```python
from build123d import *

# Parameters (mm, degrees)
BOSS_EXTRUDE2_DEPTH      = 7.35
BOSS_EXTRUDE2_DEPTH_BACK = 7.35
SKETCH2_W                = 15.7
SKETCH2_H                = 15.7
SKETCH3_R                = 8
BOSS_EXTRUDE3_DEPTH      = 20.55
SKETCH4_R                = 7.55
BOSS_EXTRUDE4_DEPTH      = 25.9
BOSS_EXTRUDE5_DEPTH      = 10
SKETCH6_R                = 8
BOSS_EXTRUDE6_DEPTH      = 20.55


with BuildPart() as part:
    # Sketch2 → Boss-Extrude2 (new, two sides: drawn at the far end of the back side and taken through both)
    with BuildSketch(Plane(origin=(0, 0, 0), x_dir=(1, 0, 0), z_dir=(0, 1, 0)).offset(-BOSS_EXTRUDE2_DEPTH_BACK)):
        Rectangle(SKETCH2_W, SKETCH2_H)
    extrude(amount=BOSS_EXTRUDE2_DEPTH + BOSS_EXTRUDE2_DEPTH_BACK)

    # Sketch3 → Boss-Extrude3 (add)
    with BuildSketch(Plane(origin=(7.85, 0, 0), x_dir=(0, 0, -1), z_dir=(1, 0, 0))):
        with Locations(Location((-0.75, 0, 0), (0, 0, 152.560759849))):
            Circle(SKETCH3_R)
    extrude(amount=BOSS_EXTRUDE3_DEPTH)

    # Sketch4 → Boss-Extrude4 (add)
    with BuildSketch(Plane(origin=(0, 0, -7.85), x_dir=(-1, 0, 0), z_dir=(0, 0, -1))):
        with Locations(Location((0, 0, 0), (0, 0, 103.217293988))):
            Circle(SKETCH4_R)
    extrude(amount=BOSS_EXTRUDE4_DEPTH)

    # Sketch5 → Boss-Extrude5 (add)
    with BuildSketch(Plane(origin=(0, 0, -33.75), x_dir=(-1, 0, 0), z_dir=(0, 0, -1))):
        Polygon((-15.532193585, 0), (-10.572107213, -10.198544939), (25.717504309, -7.313596743), (28.4, 0), (25.717504309, 7.313596743), (-10.572107213, 10.198544939), align=None)
    extrude(amount=-BOSS_EXTRUDE5_DEPTH)

    # Sketch6 → Boss-Extrude6 (add)
    with BuildSketch(Plane.XY.offset(7.85)):
        with Locations(Location((0, 0, 0), (0, 0, 168.887310083))):
            Circle(SKETCH6_R)
    extrude(amount=BOSS_EXTRUDE6_DEPTH)


solid = part.part
```
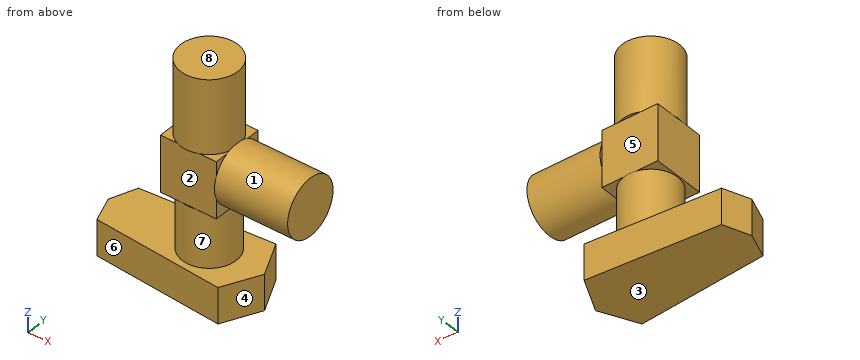
Verification items for the finished model (mm, model axes). Face numbers are marked on the shaded views. A direction names the side the tool comes from. Coordinates: 2 decimals unless noted, no trailing zeros. Loops run counter-clockwise (first coordinate to the right, second up) from the corner with the lowest first, then second, coordinate; pieces in that order, holes last. Notation, with made-up numbers: (-37.75, 80.5) -> (6.25, 80.5) arc R29 ccw to (6.25, 109.5) -> close; hole circle Ø2 at (-34, 26.25). An arc over 180 degrees is marked (long way). Put each result on its own line as item: value.
1. Gauge pin test, flat ends, axial feed: P1, Ø2, axis at x = 11, z = 1.5, coming from the -Y side; P2, Ø12, axis at y = 2, z = 2.5, coming from the -X side; P3, Ø10, axis at x = 19, z = -6.5, coming from the -Y side; P4, Ø8, axis at y = 3, z = -7.5, coming from the +X side. Record the tip position at first contact, or that the pin passes through.
Result set:
P1: stops at y = -8
P2: stops at x = -8
P3: stops at y = -7.68
P4: stops at x = 28.4
2. Section check D-D, the plane z = 13.5. Record the boundary of the cut face in (x, y).
Result set:
outline: circle Ø16 at (0, 0)
3. Mould release check, pull along Z, two halves, no side actions. Record for the marked faces 6, 7 and 8: pulls with the +Z half, pulls with the -Z half, needs draft (parallel to the pull), parting line crosses it, or undercut.
Result set:
face 6: needs draft
face 7: undercut
face 8: pulls with the +Z half
4. Section check C-C, the plane y = 8.75. Record the boundary of the cut face in (x, z).
Result set:
outline: (-7.65, -33.75) -> (11.28, -33.75) -> (11.28, -23.75) -> (-7.65, -23.75) -> close
5. Tool access check on the marked faces 1, 2, 3, 4 and 5. Record the directions out of +Z, -Z, +X, -X, +Y, -Y that give a thin tool (end or side, any length) a straight path to the whole face; none if there is none.
Result set:
face 1: +X
face 2: -X, -Y
face 3: -Z, +X, -X, +Y, -Y
face 4: -Z, +X, -Y
face 5: -X, +Y
6. Section check A-A, the plane z = 0.75. Record the boundary of the cut face in (x, y).
Result set:
outline: (-7.85, -7.35) -> (7.85, -7.35) -> (7.85, -8) -> (28.4, -8) -> (28.4, 8) -> (7.85, 8) -> (7.85, 7.35) -> (-7.85, 7.35) -> close
7. Thickness scan on line 1 (X direction, y = -3.25, z = -6.5); line 2 (Z direction, x = 6, y = 7.75); line 3 (Y direction, x = -0.5, z = -17.5). Record the ranges inside material, lowest first.
Result set:
line 1: x = -7.85 to 28.4
line 2: z = -33.75 to -23.75
line 3: y = -7.53 to 7.53
8. Section check B-B, the plane x = 0. Record the boundary of the cut face in (y, z), then the cut area to 3 significant figures.
Result set:
outline: (-9.36, -33.75) -> (9.36, -33.75) -> (9.36, -23.75) -> (7.55, -23.75) -> (7.55, -7.85) -> (7.35, -7.85) -> (7.35, 7.85) -> (8, 7.85) -> (8, 28.4) -> (-8, 28.4) -> (-8, 7.85) -> (-7.35, 7.85) -> (-7.35, -7.85) -> (-7.55, -7.85) -> (-7.55, -23.75) -> (-9.36, -23.75) -> close
area: 987 mm^2
